Autodesk Inventor part; units mm, degrees
ref_plane "YZ Plane" through (0, 0, 0) normal (1, 0, 0) x (0, 1, 0)
ref_plane "XZ Plane" through (0, 0, 0) normal (0, 1, 0) x (-1, 0, 0)
ref_plane "XY Plane" through (0, 0, 0) normal (0, 0, 1) x (1, 0, 0)
sketch "Boceto1" plane through (0, 0, 0) normal (0, 0, 1) x (1, 0, 0)
  line L0 (-508.547, 495.7265) -> (491.453, 495.7265)
  line L1 (491.453, 495.7265) -> (491.453, -4.2735)
  line L2 (491.453, -4.2735) -> (-508.547, -4.2735)
  line L3 (-508.547, -4.2735) -> (-508.547, 495.7265)
  line L4 (-458.547, 445.7265) -> (441.453, 445.7265)
  line L5 (441.453, 45.7265) -> (-458.547, 45.7265)
  line L6 (441.453, 270.7265) -> (-458.547, 270.7265)
  line L7 (-458.547, 220.7265) -> (441.453, 220.7265)
  line L8 (-458.547, 270.7265) -> (-458.547, 445.7265)
  line L9 (-458.547, 220.7265) -> (-458.547, 45.7265)
  line L10 (441.453, 270.7265) -> (441.453, 445.7265)
  line L11 (441.453, 220.7265) -> (441.453, 45.7265)
  point P0 (0, 0)
  dimension "d0" = 1000
  dimension "d1" = 500
  dimension "d2" = 900
  dimension "d4" = 400
  dimension "d5" = 50
  dimension "d17" = 175
  dimension "d18" = 175
  dimension "d19" = 175
  dimension "d20" = 175
extrude "Extrusión1" add sketch "Boceto1" along normal blind 50
properties part number "Base_mesa" material "Hierro, fundido"
Design review of the part built by this model. Coordinates are the model's own, in mm. A direction names the side the tool comes from. Give positions to 0.01 mm unless a question says otherwise; leave off trailing zeros. Write each loop counter-clockwise with the first axis right and the second up, starting at its lowest first coordinate (ties: lowest second). Pieces come first, ordered by that corner, then holes.
(1) Add section B-B (x = -366.5). Give the boundary of the cut face in (y, z), and give its area (3 significant figures).
Checked values:
outline: (-4.27, 0) - (45.73, 0) - (45.73, 50) - (-4.27, 50) - close; (220.73, 0) - (270.73, 0) - (270.73, 50) - (220.73, 50) - close; (445.73, 0) - (495.73, 0) - (495.73, 50) - (445.73, 50) - close
area: 7,500 mm2
(2) Add section A-A (y = 431.5). Give the boundary of the cut face in (x, z), and give its area (3 significant figures).
Checked values:
outline: (-508.55, 0) - (-458.55, 0) - (-458.55, 50) - (-508.55, 50) - close; (441.45, 0) - (491.45, 0) - (491.45, 50) - (441.45, 50) - close
area: 5,000 mm2
(3) Tool access review of faces 4 (the face through (-2, 270.726, 25)), 5 (the face through (-508.547, 242, 25)): name each direction out of +Z, -Z, +X, -X, +Y, -Y from which nothing blocks a thin tool from reaching the whole face with its end or side.
Checked values:
face 4: +Z, -Z
face 5: +Z, -Z, -X, +Y, -Y
(4) Add section C-C (z = 10.5). Give the boundary of the cut face in (x, y), and give its area (3 significant figures).
Checked values:
outline: (-508.55, -4.27) - (491.45, -4.27) - (491.45, 495.73) - (-508.55, 495.73) - close; hole (-458.55, 45.73) - (441.45, 45.73) - (441.45, 220.73) - (-458.55, 220.73) - close; hole (-458.55, 270.73) - (441.45, 270.73) - (441.45, 445.73) - (-458.55, 445.73) - close
area: 185,000 mm2
(5) Mouldability with a two-part tool opening along Y and no side actions: class faces 1 (the face through (-458.547, 134, 25)), 2 (the face through (-127, 249, 50)), 3 (the face through (-2, -4.274, 25)) as +Y half, -Y half, draft (parallel to the pull), parting line (faces both ways), or undercut.
Checked values:
face 1: undercut
face 2: draft
face 3: -Y half
(6) Wall thickness on line 1 along Y through (x, z) = (231.5, 18.5); line 2 along X through (y, z) = (371, 38.5): over which ranges is each line inside the solid? List them lowest first.
Checked values:
line 1: y = -4.27 to 45.73, 220.73 to 270.73, 445.73 to 495.73
line 2: x = -508.55 to -458.55, 441.45 to 491.45
